The model under review builds one solid part; all positions refer to its coordinate system, in mm. A direction names the side the tool comes from. Give positions to 0.01 mm unless a question says otherwise; leave off trailing zeros. Loops run counter-clockwise (first coordinate to the right, second up) from the corner with the lowest first, then second, coordinate; pieces in that order, holes last. Notation, with made-up numbers: M 33,89.5 L 52,89.5 A23 cw 52,124.5 Z; hole C 63.5,67.5 d8. An arc over 180 degrees is marked long. Put each result on its own line as item: value. Start each with the question number.
```python
from build123d import *

# Parameters (mm, degrees)
SKETCH1_W             = 40.5
SKETCH1_H             = 20
BOSS_EXTRUDE1_DEPTH   = 39.1
SKETCH2_R             = 6.75
BOSS_EXTRUDE2_DEPTH   = 2.1
SKETCH3_R             = 4.25
BOSS_EXTRUDE3_DEPTH   = 6.4
SKETCH4_W             = 2.5
SKETCH4_H             = 20
BOSS_EXTRUDE4_DEPTH   = 7.5
CHAMFER1_SIZE2        = 7.5
CHAMFER1_SIZE         = 1.5
CUT_EXTRUDE1_DEPTH    = 9.5
CHAMFER2_SIZE2        = 7.5
CHAMFER2_SIZE         = 1.5
MIRROR19_COPY_1_DEPTH = 9.5


with BuildPart() as part:
    # Sketch1 → Boss-Extrude1 (new body)
    with BuildSketch(Plane.XY):
        with Locations((20.25, 10)):
            Rectangle(SKETCH1_W, SKETCH1_H)
    extrude(amount=BOSS_EXTRUDE1_DEPTH)

    # Sketch2 → Boss-Extrude2 (add)
    with BuildSketch(Plane.XY.offset(39.1)):
        with Locations(Location((9.75, 10, 0), (0, 0, 180))):
            Circle(SKETCH2_R)
    extrude(amount=BOSS_EXTRUDE2_DEPTH)

    # Sketch3 → Boss-Extrude3 (add)
    with BuildSketch(Plane.XY.offset(41.2)):
        with Locations((9.75, 10)):
            Circle(SKETCH3_R)
    extrude(amount=BOSS_EXTRUDE3_DEPTH)

    # Sketch4 → Boss-Extrude4 (add)
    with BuildSketch(Plane(origin=(40.5, 0, 0), x_dir=(0, 0, -1), z_dir=(1, 0, 0))):
        with Locations((-28.55, 10)):
            Rectangle(SKETCH4_W, SKETCH4_H)
    boss_extrude4 = extrude(amount=BOSS_EXTRUDE4_DEPTH)

    # Chamfer1
    chamfer1_edges = [part.edges().sort_by_distance(p)[0] for p in [
        (40.5, 10, 29.8),
    ]]
    chamfer1_side = [part.faces().sort_by_distance(p)[0] for p in [
        (40.5, 10, 29.83),
    ]]
    chamfer(chamfer1_edges, length=CHAMFER1_SIZE - 0.0001, length2=CHAMFER1_SIZE2 - 0.0001, reference=chamfer1_side[0])  # a hair under: the kernel refuses the full size

    # Sketch5 → Cut-Extrude1 (cut)
    with BuildSketch(Plane.XZ):
        Polygon((48, 29.8), (40.5, 29.8), (40.5, 31.3), align=None)
    cut_extrude1 = extrude(amount=-CUT_EXTRUDE1_DEPTH, mode=Mode.SUBTRACT)

    # Mirror1: Cut-Extrude1 across plane
    add(cut_extrude1.mirror(Plane.ZX.offset(10)), mode=Mode.SUBTRACT)

    # Mirror11: Boss-Extrude4 across plane
    add(boss_extrude4.mirror(Plane(origin=(20.25, 0, 0), x_dir=(0, 0, 1), z_dir=(1, 0, 0))))

    # Chamfer2
    chamfer2_edges = [part.edges().sort_by_distance(p)[0] for p in [
        (0, 10, 29.8),
    ]]
    chamfer2_side = [part.faces().sort_by_distance(p)[0] for p in [
        (0, 10, 29.83),
    ]]
    chamfer(chamfer2_edges, length=CHAMFER2_SIZE - 0.0001, length2=CHAMFER2_SIZE2 - 0.0001, reference=chamfer2_side[0])  # a hair under: the kernel refuses the full size

    # Mirror19: Cut-Extrude1 across plane
    add(cut_extrude1.mirror(Plane(origin=(20.25, 0, 0), x_dir=(0, 0, 1), z_dir=(1, 0, 0))), mode=Mode.SUBTRACT)

    # Mirror19 copy 1 sketch → Mirror19 copy 1 (cut)
    with BuildSketch(Plane(origin=(40.5, 20, 0), x_dir=(-1, 0, 0), z_dir=(0, 1, 0))):
        Polygon((48, 29.8), (40.5, 29.8), (40.5, 31.3), align=None)
    extrude(amount=-MIRROR19_COPY_1_DEPTH, mode=Mode.SUBTRACT)


solid = part.part
```
Item 1: Clearance check with flat-ended pins moving along their axes: pin 1 Ø8 at (x, y) = (42.5, 14.5) entering from +Z; pin 2 Ø2 at (x, y) = (-3.5, 13) entering from +Z; pin 3 Ø1 at (y, z) = (13.5, 15.5) entering from +X. State where each tip first meets the part, or that it passes through.
Item 2: Consider section A-A, the plane x = 9.75. Write out the cut boundary in (y, z), plus the area to 3 significant figures.
Item 3: To check wall thickness, follow L1, parallel to X at y = 7.5, z = 2; L2, parallel to Z at x = 5.5, y = 8; L3, parallel to Z at x = 20.5, y = 13. State the ranges of each line that lie inside material, in increasing order. Write a range as [from, to].
Item 4: Tool access review of faces 1 (the flat face through (40.5, 10, 13)), 2 (the flat face through (-4, 10, 27.3)), 3 (the flat face through (43, 10.5, 30)), 4 (the flat face through (44, 8, 29.8)), 5 (the flat face through (43, 9.5, 30)): name each direction out of +Z, -Z, +X, -X, +Y, -Y from which nothing blocks a thin tool from reaching the whole face with its end or side.
Item 5: Consider section B-B, the plane y = 6.5. Write out the cut boundary in (x, z).
Item 6: Consider section C-C, the plane z = 13.5. Write out the cut boundary in (x, y), plus the area to 3 significant figures.
Item 7: Consider section D-D, the plane x = 18. Write out the cut boundary in (y, z), plus the area to 3 significant figures.
Report:
1. pin 1: z = 39.1
1. pin 2: z = 29.8
1. pin 3: x = 40.5
2. outline: M 0,0 L 20,0 L 20,39.1 L 16.75,39.1 L 16.75,41.2 L 14.25,41.2 L 14.25,47.6 L 5.75,47.6 L 5.75,41.2 L 3.25,41.2 L 3.25,39.1 L 0,39.1 Z
2. area: 865 mm²
3. L1: [0, 40.5]
3. L2: [0, 41.2]
3. L3: [0, 39.1]
4. face 1: -Z, +X, +Y, -Y
4. face 2: -Z, -X, +Y, -Y
4. face 3: +Z, +X, +Y
4. face 4: +Z, +X, -Y
4. face 5: +Z, +X, -Y
5. outline: M -7.5,27.3 L 0,27.3 L 0,0 L 40.5,0 L 40.5,27.3 L 48,27.3 L 48,29.8 L 40.5,29.8 L 40.5,39.1 L 15.52,39.1 L 15.52,41.2 L 12.16,41.2 L 12.16,47.6 L 7.34,47.6 L 7.34,41.2 L 3.98,41.2 L 3.98,39.1 L 0,39.1 L 0,29.8 L -7.5,29.8 Z
6. outline: M 0,0 L 40.5,0 L 40.5,20 L 0,20 Z
6. area: 810 mm²
7. outline: M 0,0 L 20,0 L 20,39.1 L 0,39.1 Z
7. area: 782 mm²
